Input: part model. Units: mm. Frame: model coordinates. Face numbers are marked on the shaded views. A direction names the side the tool comes from. Give positions to 0.01 mm unless a question says otherwise; leave off trailing zeros. Loops run counter-clockwise (first coordinate to the right, second up) from the corner with the lowest first, then second, coordinate; pieces in that order, holes last. Notation, with made-up numbers: (62.25, -33) - (106.25, -33) arc R31 cw to (106.25, -3) - close; hole circle Ø4 at (80, -34). An arc over 180 degrees is marked (long way). One line per question, with ' | ' between items. Start each with the question number.
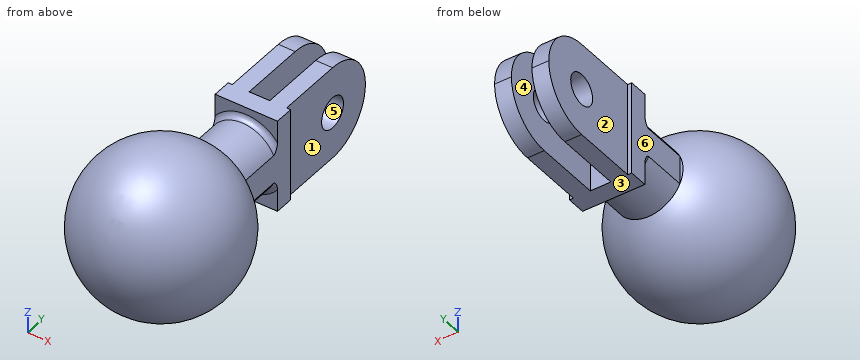
from build123d import *

# Parameters (mm, degrees)
SKETCH2_W           = 10
SKETCH2_H           = 15
BOSS_EXTRUDE1_DEPTH = 3
SKETCH3_W           = 2.7
SKETCH3_H           = 15
BOSS_EXTRUDE2_DEPTH = 18
SKETCH4_R           = 2.5
CUT_EXTRUDE1_DEPTH  = 39.541399757
SKETCH5_W           = 3.267109453
SKETCH5_H           = 13.055369116
SKETCH5_W_2         = 2.399629859
SKETCH5_H_2         = 12.441962392
CUT_EXTRUDE2_DEPTH  = 11


with BuildPart() as part:
    # Sketch1 → Revolve1 (revolve)
    with BuildSketch(Plane.XY, mode=Mode.PRIVATE) as revolve1_sk:
        with BuildLine():
            Line((5.5, 0), (0, 0))
            Line((0, 0), (0, -32.147270417))
            ThreePointArc((0, -32.147270417), (12.382857794, -22.267701741), (5.5, -8))
            Line((5.5, -8), (5.5, -0.86171942))
            Line((5.5, -0.86171942), (5.5, 0))
        make_face()
        with BuildLine():
            Line((6.36171942, 0), (5.5, 0))
            Line((5.5, 0), (5.5, -0.86171942))
            ThreePointArc((5.5, -0.86171942), (5.77082934, -0.27082934), (6.36171942, 0))
        make_face()
    revolve(revolve1_sk.sketch.rotate(Axis((0, 0, 0), (0, -1, 0)), 90), axis=Axis((0, 0, 0), (0, -1, 0)))

    # Sketch2 → Boss-Extrude1 (add)
    with BuildSketch(Plane(origin=(0, 0, 0), x_dir=(1, 0, 0), z_dir=(0, 1, 0))):
        Rectangle(SKETCH2_W, SKETCH2_H)
    extrude(amount=BOSS_EXTRUDE1_DEPTH)

    # Sketch3 → Boss-Extrude2 (add)
    with BuildSketch(Plane(origin=(0, 3, 0), x_dir=(1, 0, 0), z_dir=(0, 1, 0))):
        with Locations((-3, 0)):
            Rectangle(SKETCH3_W, SKETCH3_H)
        with Locations((3, 0)):
            Rectangle(SKETCH3_W, SKETCH3_H)
    extrude(amount=BOSS_EXTRUDE2_DEPTH)

    # Sketch4 → Cut-Extrude1 (cut, through all)
    with BuildSketch(Plane.ZY.offset(4.35)):
        with Locations((0, 13.5)):
            Circle(SKETCH4_R)
        with BuildLine():
            Line((-7.5, 21), (-7.5, 13.5))
            ThreePointArc((-7.5, 13.5), (-5.303300859, 18.803300859), (0, 21))
            Line((0, 21), (-7.5, 21))
        make_face()
        with BuildLine():
            Line((7.5, 21), (0, 21))
            ThreePointArc((0, 21), (5.303300859, 18.803300859), (7.5, 13.5))
            Line((7.5, 13.5), (7.5, 21))
        make_face()
    extrude(amount=-CUT_EXTRUDE1_DEPTH, mode=Mode.SUBTRACT)

    # Sketch5 → Cut-Extrude2 (cut)
    with BuildSketch(Plane(origin=(0, 3, 0), x_dir=(1, 0, 0), z_dir=(0, 1, 0))):
        with Locations((6.633554726, 0.972315442)):
            Rectangle(SKETCH5_W, SKETCH5_H)
        with Locations((-6.19981493, 1.279018804)):
            Rectangle(SKETCH5_W_2, SKETCH5_H_2)
    extrude(amount=-CUT_EXTRUDE2_DEPTH, mode=Mode.SUBTRACT)


solid = part.part
Q1. Section C-C, the plane z = -11. Output: boundary loops of the cut face in (x, y), plus the area to 3 significant figures.
Q2. Line query: L1, parallel to X at y = 5.5, z = 6.25; L2, parallel to X at y = 1, z = -3.5. Output: solid intervals per line, ascending. Write a range as from..to.
Q3. Section A-A, the plane y = 5.5. Output: boundary loops of the cut face in (x, z).
Q4. Draft query along Y for the marked faces 5 and 6. Return one class per face: +Y half, -Y half, draft (parallel to the pull), parting line (faces both ways), or undercut.
Q5. Section D-D, the plane x = 8.25. Output: boundary loops of the cut face in (y, z), plus the area to 3 significant figures.
Q6. Section B-B, the plane y = -5. Output: boundary loops of the cut face in (x, z), plus the area to 3 significant figures.
Q7. Access query for the marked faces 1, 2, 3 and 4. Directions: +Z, -Z, +X, -X, +Y, -Y. A direction counts if a zero-diameter tool reaches every point of the face in a straight line with its end or side. Return the directions, or none.
Q8. First-contact query: pin 1 (8 mm diameter, centred on x = 10, z = -4, fed in from -Y); pin 2 (6 mm diameter, centred on y = -26.5, z = -5.5, fed in from -X); pin 3 (8 mm diameter, centred on y = 13.5, z = 0, fed in from +X). Flat tips, straight axial feed; report the tip coordinate or a pass-through.
Solved:
1) outline: circle Ø12.69 at (0, -19.45) | area: 127 mm²
2) L1: x = -4.35..-1.65, 1.65..4.35 | L2: x = -5..5
3) outline: (-4.35, -7.5) - (-1.65, -7.5) - (-1.65, 7.5) - (-4.35, 7.5) - close; (1.65, -7.5) - (4.35, -7.5) - (4.35, 7.5) - (1.65, 7.5) - close
4) face 5: undercut | face 6: draft
5) outline: circle Ø19.31 at (-19.45, 0) | area: 293 mm²
6) outline: (-5, -2.29) arc R5.5 ccw to (5, -2.29) - (5, 2.29) arc R5.5 ccw to (-5, 2.29) - close | area: 91.9 mm²
7) face 1: +Z, -Z, +X, +Y | face 2: +Z, -Z, -X, +Y | face 3: -Z, +X, -X, +Y | face 4: +Z, -Z, +Y
8) pin 1: stops at y = -30.19 | pin 2: stops at x = -11.22 | pin 3: stops at x = 4.35
